Design review of the part built by this model. Coordinates are the model's own, in mm. A direction names the side the tool comes from. Give positions to 0.01 mm unless a question says otherwise; leave off trailing zeros. Order: outer loops, then holes, each group sorted by start corner. A loop starts at its lowest first (then second) coordinate and runs counter-clockwise, first axis right, second up. Notation, with made-up numbers: (74.5, -35) -> (106.5, -35) arc R22 ccw to (106.5, -7) -> close; hole circle Ø1 at (85, 63). An arc over 180 degrees is marked (long way). One line per item, written item: value. Start each with the question number.
1) Consider section A-A (z = 38.1). State the section outline as (x, y) points.
2) Tool access review of faces 1 (the face through (6.261, -0.477, -19.413)), 2 (the face through (12.7, 0.1, -57.5)), 3 (the face through (11.23, -31.66, 54.47)): name each direction out of +Z, -Z, +X, -X, +Y, -Y from which nothing blocks a thin tool from reaching the whole face with its end or side.
3) Wall thickness on line 1 along Z through (x, y) = (13, -0.5); line 2 along Y through (x, z) = (14.5, 38.1); line 3 along Z through (x, y) = (16, 4): over which ranges is each line inside the solid? List them lowest first. Write a range as from..to.
4) The part is to be moulded in two halves that separate along X. For faces 4 (the face through (12.7, -2, 38)), 5 (the face through (9.019, -23.797, -0.022)), 6 (the face through (9.151, -23.797, 56.807)), 7 (the face through (6.261, -0.477, 39.614)), say which applies: released by +X, released by -X, zero draft, split by the parting line, or undercut.
5) For pin 1 (5 mm diameter, centred on y = 0.5, z = 38, fed in from +X); pin 2 (3 mm diameter, centred on y = 0, z = 13.55, fed in from -X); pin 3 (4 mm diameter, centred on x = 9.525, z = -63.5, fed in from -Y), all flat-tipped, find the tip position at first contact; note any pin that passes through.
from build123d import *

# Parameters (mm, degrees)
SKETCH1_W           = 152.4
SKETCH1_H           = 76.2
SKETCH1_R           = 1.5875
SKETCH1_R_2         = 1.190625
BOSS_EXTRUDE1_DEPTH = 19.05
SKETCH3_R           = 4.7625
CUT_EXTRUDE2_DEPTH  = 6.35


with BuildPart() as part:
    # Sketch1 → Boss-Extrude1 (new body)
    with BuildSketch(Plane(origin=(0, 0, 0), x_dir=(0, 0, -1), z_dir=(1, 0, 0))):
        Rectangle(SKETCH1_W, SKETCH1_H)
        with Locations(Location((-38.1, 0, 0), (0, 0, 180))):
            Circle(SKETCH1_R, mode=Mode.SUBTRACT)
        with Locations(Location((-13.55, 0, 0), (0, 0, 180))):
            Circle(SKETCH1_R, mode=Mode.SUBTRACT)
        with Locations(Location((20.927, 0, 0), (0, 0, 180))):
            Circle(SKETCH1_R, mode=Mode.SUBTRACT)
        with Locations(Location((55.404, 0, 0), (0, 0, 180))):
            Circle(SKETCH1_R, mode=Mode.SUBTRACT)
        with Locations(Location((-63.5, -0.396875, 0), (0, 0, 180))):
            Circle(SKETCH1_R_2, mode=Mode.SUBTRACT)
        with Locations(Location((-63.5, 3.175, 0), (0, 0, 180))):
            Circle(SKETCH1_R, mode=Mode.SUBTRACT)
    extrude(amount=BOSS_EXTRUDE1_DEPTH)

    # Sketch3 → Cut-Extrude2 (cut)
    with BuildSketch(Plane(origin=(19.05, 0, 0), x_dir=(0, 0, -1), z_dir=(1, 0, 0))):
        with Locations((-38.1, 0)):
            Circle(SKETCH3_R)
        with Locations((-13.55, 0)):
            Circle(SKETCH3_R)
        with Locations((20.927, 0)):
            Circle(SKETCH3_R)
        with Locations((55.404, 0)):
            Circle(SKETCH3_R)
    extrude(amount=-CUT_EXTRUDE2_DEPTH, mode=Mode.SUBTRACT)

    # 1/4 (0.25) Diameter Hole1: read off the stored shape, not the designer's step
    # 1/4 (0.25) Diameter Hole1 outline → 1/4 (0.25) Diameter Hole1 (revolve, cut)
    with BuildSketch(Plane(origin=(9.525, 0, 57.15), x_dir=(1, 0, 0), z_dir=(0, 0, 1))):
        Polygon((3.175, -25.4), (0, -23.492267535), (0, -38.1), (3.175, -38.1), align=None)
    revolve(axis=Axis((9.525, 0, 57.15), (0, 1, 0)), mode=Mode.SUBTRACT)

    # 1_4 _0.25_ Diameter Hole1 2 outline → 1_4 _0.25_ Diameter Hole1 2 (revolve, cut)
    with BuildSketch(Plane(origin=(9.525, 0, 0), x_dir=(1, 0, 0), z_dir=(0, 0, 1))):
        Polygon((3.175, -25.4), (0, -23.492267535), (0, -38.1), (3.175, -38.1), align=None)
    revolve(axis=Axis((9.525, 0, 0), (0, 1, 0)), mode=Mode.SUBTRACT)

    # 1_4 _0.25_ Diameter Hole1 3 outline → 1_4 _0.25_ Diameter Hole1 3 (revolve, cut)
    with BuildSketch(Plane(origin=(9.525, 0, -63.5), x_dir=(1, 0, 0), z_dir=(0, 0, 1))):
        Polygon((3.175, -25.4), (0, -23.492267535), (0, -38.1), (3.175, -38.1), align=None)
    revolve(axis=Axis((9.525, 0, -63.5), (0, 1, 0)), mode=Mode.SUBTRACT)


solid = part.part
Checked values:
1. outline: (0, -38.1) -> (19.05, -38.1) -> (19.05, -4.76) -> (12.7, -4.76) -> (12.7, -1.59) -> (0, -1.59) -> close; (0, 1.59) -> (12.7, 1.59) -> (12.7, 4.76) -> (19.05, 4.76) -> (19.05, 38.1) -> (0, 38.1) -> close
2. face 1: +X, -X
2. face 2: +X
2. face 3: -Y
3. line 1: z = -76.2..-60.14, -50.67..-25.66, -16.19..8.81, 18.29..33.36, 42.84..62.31, 64.69..76.2
3. line 2: y = -38.1..-4.76, 4.76..38.1
3. line 3: z = -76.2..-57.99, -52.82..-23.51, -18.34..10.97, 16.13..35.52, 40.68..62.14, 64.86..76.2
4. face 4: released by +X
4. face 5: undercut
4. face 6: undercut
4. face 7: zero draft
5. pin 1: stops at x = 12.7
5. pin 2: passes through
5. pin 3: stops at y = -24.69
